Can you work these out from the drawing? Everything is in mm from the part's minimum corner. A direction names the side the tool comes from. Coordinates: 2 decimals unless noted, no trailing zeros. Loops run counter-clockwise (first coordinate to the right, second up) from the corner with the lowest first, then second, coordinate; pieces in that order, holes last. Notation, with made-up numbers: (11, -36.75) - (46, -36.75) arc R29 cw to (46, -3.75) - close; hole circle Ø5 at (71.5, 13.5). An arc over 180 degrees is marked (long way). One line per question, with ' | ' between items. Start each with the question number.
1. Which directions (+Z, -Z, +X, -X, +Y, -Y) give clear straight access to the entire face, cutting with the end or side of a thin tool? Please do the marked faces 1, 2, 3, 4 and 5.
2. I want a section at A-A, the plane x = 57.5. Write out the boundary of the cut face in (y, z) (1 decimal).
3. I want a section at C-C, the plane z = 33.5. Write out the boundary of the cut face in (x, y).
4. I want a section at B-B, the plane y = 9.5. Write out the boundary of the cut face in (x, z) (1 decimal).
5. Please list where these lines run through material, in increasing order: L1, parallel to Y at x = 60, z = 25.5; L2, parallel to Y at x = 12, z = 115.5; L3, parallel to X at y = 101, z = 28. Write a range as [from, to].
6. I'm going to push flat-ended pins straight in: P1, Ø8, axis at y = 45.5, z = 17, coming from the -X side; P2, Ø20.5, axis at x = 53, z = 18.5, coming from the -Y side; P3, Ø8, axis at y = 99.5, z = 73, coming from the -X side. Where does each tip first touch, or does it pass through?
7. I want a section at D-D, the plane x = 23. Write out the boundary of the cut face in (y, z) (1 decimal).
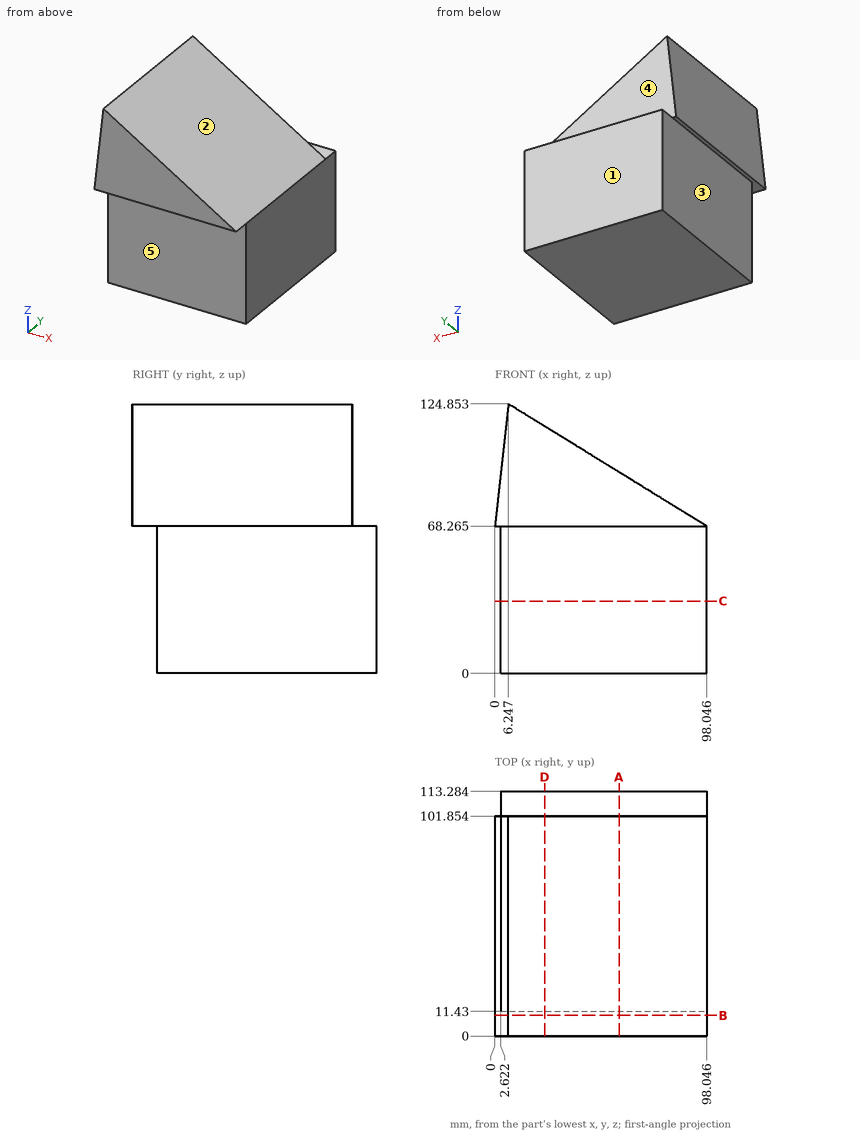
Results are:
1) face 1: +Z, -Z, +X, -X, +Y | face 2: +Z, +X, +Y, -Y | face 3: -Z, -X, +Y, -Y | face 4: +Z, +X, -X, +Y | face 5: -Z, +X, -X, -Y
2) outline: (0, 68.3) - (11.4, 68.3) - (11.4, 0) - (113.3, 0) - (113.3, 68.3) - (101.9, 68.3) - (101.9, 93.3) - (0, 93.3) - close
3) outline: (2.62, 11.43) - (98.05, 11.43) - (98.05, 113.28) - (2.62, 113.28) - close
4) outline: (0, 68.3) - (98, 68.3) - (6.2, 124.9) - close
5) L1: y = [11.43, 113.28] | L2: y = [0, 101.85] | L3: x = [2.62, 98.05]
6) P1: stops at x = 2.62 | P2: stops at y = 11.43 | P3: stops at x = 0.08
7) outline: (0, 68.3) - (11.4, 68.3) - (11.4, 0) - (113.3, 0) - (113.3, 68.3) - (101.9, 68.3) - (101.9, 114.5) - (0, 114.5) - close
